The model under review builds one solid part; all positions refer to its coordinate system, in mm. A direction names the side the tool comes from. Round coordinates to 2 decimals unless told otherwise and drop trailing zeros. Loops run counter-clockwise (first coordinate to the right, second up) from the corner with the lowest first, then second, coordinate; pieces in that order, holes last. Notation, with made-up numbers: M 3,46.25 L 9,46.25 A25 cw 9,72.25 Z; hole C 77,-33 d9. An arc over 180 degrees is marked long. One line per question, with ' | ' between items.
from build123d import *

# Parameters (mm, degrees)
SKETCH1_W           = 10.9982
SKETCH1_H           = 5.588
BOSS_EXTRUDE1_DEPTH = 5.0038
SKETCH2_W           = 6.604
SKETCH2_H           = 3.4036
CUT_EXTRUDE1_DEPTH  = 0.254
SKETCH3_W           = 3.4036
SKETCH3_H           = 3.2004
BOSS_EXTRUDE2_DEPTH = 5.2578
SKETCH4_W           = 0.8128
SKETCH4_H           = 0.508
BOSS_EXTRUDE3_DEPTH = 4.318
LPATTERN1_COUNT     = 2
LPATTERN1_PITCH     = 3.2004
LPATTERN1_COL_COUNT = 2
LPATTERN1_COL_PITCH = 3.2004


with BuildPart() as part:
    # Sketch1 → Boss-Extrude1 (new body)
    with BuildSketch(Plane(origin=(0, 0, 0), x_dir=(1, 0, 0), z_dir=(0, 1, 0))):
        Rectangle(SKETCH1_W, SKETCH1_H)
    extrude(amount=BOSS_EXTRUDE1_DEPTH)

    # Sketch2 → Cut-Extrude1 (cut)
    with BuildSketch(Plane(origin=(0, 5.0038, 0), x_dir=(1, 0, 0), z_dir=(0, 1, 0))):
        Rectangle(SKETCH2_W, SKETCH2_H)
    extrude(amount=-CUT_EXTRUDE1_DEPTH, mode=Mode.SUBTRACT)

    # Sketch3 → Boss-Extrude2 (add)
    with BuildSketch(Plane(origin=(0, 4.7498, 0), x_dir=(1, 0, 0), z_dir=(0, 1, 0))):
        with Locations((-1.59766, 0)):
            Rectangle(SKETCH3_W, SKETCH3_H)
    extrude(amount=BOSS_EXTRUDE2_DEPTH)

    # Sketch4 → Boss-Extrude3 (add)
    with BuildSketch(Plane.XZ):
        Rectangle(SKETCH4_W, SKETCH4_H)
    boss_extrude3 = extrude(amount=BOSS_EXTRUDE3_DEPTH)

    # LPattern1: Boss-Extrude3 ×2
    with Locations(*[(i * LPATTERN1_PITCH, 0, 0) for i in range(1, LPATTERN1_COUNT)]):
        add(boss_extrude3)

    # LPattern1 col: Boss-Extrude3 ×2
    with Locations(*[(-i * LPATTERN1_COL_PITCH, 0, 0) for i in range(1, LPATTERN1_COL_COUNT)]):
        add(boss_extrude3)


solid = part.part
1) Add section A-A on y = -3. State the section outline as (x, z) points.
Output values:
outline: M -3.61,-0.25 L -2.79,-0.25 L -2.79,0.25 L -3.61,0.25 Z; M -0.41,-0.25 L 0.41,-0.25 L 0.41,0.25 L -0.41,0.25 Z; M 2.79,-0.25 L 3.61,-0.25 L 3.61,0.25 L 2.79,0.25 Z
2) Insertion check: P1, Ø1, axis at x = -2, y = 7.5, coming from the -Z side; P2, Ø3, axis at x = -2, z = 1, coming from the -Y side; P3, Ø1, axis at x = -4, z = -1.5, coming from the -Y side; P4, Ø1, axis at x = -1.5, y = 7.5, coming from the +Z side. Each pin has a flat end and moves straight along its axis. Give the tip position at first contact, or say it passes through.
Output values:
P1: stops at z = -1.6 | P2: stops at y = -4.32 | P3: stops at y = 0 | P4: stops at z = 1.6
3) Add section D-D on x = -1.5. State the section outline as (y, z) points, then the cut area to 3 significant figures.
Output values:
outline: M 0,-2.79 L 5,-2.79 L 5,-1.7 L 4.75,-1.7 L 4.75,-1.6 L 10.01,-1.6 L 10.01,1.6 L 4.75,1.6 L 4.75,1.7 L 5,1.7 L 5,2.79 L 0,2.79 Z | area: 43.9 mm²
4) For line 1 (Y direction, x = -2.5, z = 0); line 2 (Y direction, x = -4.75, z = -0.7); line 3 (X direction, y = 8.75, z = 0.75), list the stretches that pass through material, from the lowest coordinate up.
Output values:
line 1: y = 0 to 10.01 | line 2: y = 0 to 5 | line 3: x = -3.3 to 0.1
5) Machinability: for faces 1 (the flat face through (0, -2, -0.254)), 2 (the flat face through (-3, -2, 0.254)), 3 (the flat face through (0, 2, -2.794)), which of the approach directions +Z, -Z, +X, -X, +Y, -Y give a long, thin tool a straight path to every point of the face, cutting with its end or side? Answer none if there is none.
Output values:
face 1: -Z, +X, -X, -Y | face 2: +Z, +X, -X, -Y | face 3: -Z, +X, -X, +Y, -Y
6) Mouldability with a two-part tool opening along X and no side actions: class faces 4 (the flat face through (-3, -2, -0.254)), 5 (the flat face through (-5.499, 2, 0)), 6 (the flat face through (2, 4.75, 0)) as +X half, -X half, draft (parallel to the pull), parting line (faces both ways), or undercut.
Output values:
face 4: draft | face 5: -X half | face 6: undercut
7) Add section C-C on x = -0.25. State the section outline as (y, z) points.
Output values:
outline: M -4.32,-0.25 L 0,-0.25 L 0,-2.79 L 5,-2.79 L 5,-1.7 L 4.75,-1.7 L 4.75,-1.6 L 10.01,-1.6 L 10.01,1.6 L 4.75,1.6 L 4.75,1.7 L 5,1.7 L 5,2.79 L 0,2.79 L 0,0.25 L -4.32,0.25 Z
